Check sheet for the drawn part. Datum: minimum x, y, z corner. Units: mm. A direction names the side the tool comes from. Coordinates: 2 decimals unless noted, no trailing zeros. Loops run counter-clockwise (first coordinate to the right, second up) from the corner with the lowest first, then second, coordinate; pieces in that order, holes last. Notation, with made-up numbers: M 41.5,-3.75 L 65.5,-3.75 A26 cw 65.5,24.25 Z; hole C -3,-16.5 d5. An arc over 180 degrees is marked long. Answer as CSV lines item,"result". Start each with the question number.
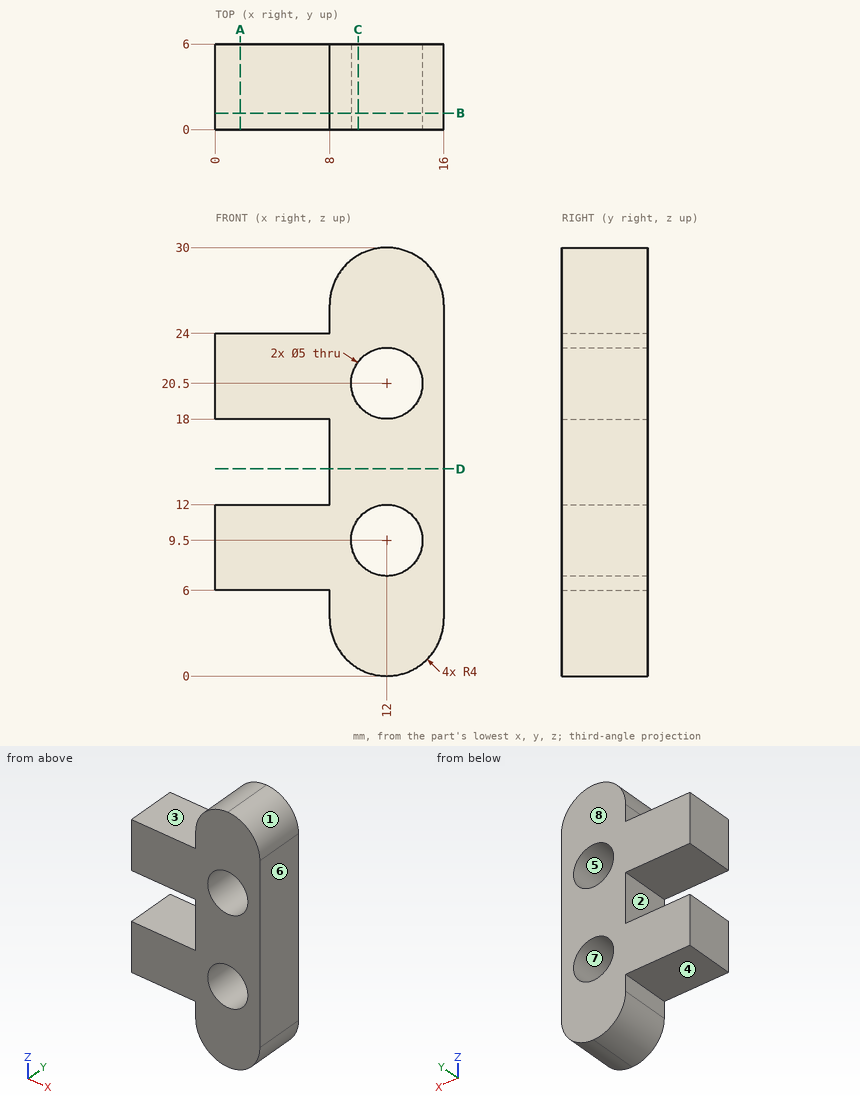
Item 1: Sectioned sample at C-C, the plane x = 10. Record the boundary of the cut face in (y, z).
Item 2: Go/stop test with flat-tipped pins: pin 1 (1.5 mm diameter, centred on y = 4.5, z = 4.5, fed in from -X); pin 2 (3 mm diameter, centred on x = 4.5, y = 1.5, fed in from +Z); pin 3 (3 mm diameter, centred on x = 5.5, y = 1.5, fed in from -Z). Record where each tip stops, or that it passes through.
Item 3: Set-up check for the marked faces 1, 2, 3 and 4: record each of +Z, -Z, +X, -X, +Y, -Y from which the full face is reachable in a straight line by a thin tool's end or side.
Item 4: Sectioned sample at B-B, the plane y = 1.15. Give the number of separate pieces and of enclosed holes in the cut face, and give its area (3 significant figures).
Item 5: Sectioned sample at D-D, the plane z = 14.5. Record the boundary of the cut face in (x, y).
Item 6: Release check for a two-part mould opening along X. For the marked faces 5, 6, 7 and 8 record: released by +X, released by -X, zero draft, split by the parting line, or undercut.
Item 7: Sectioned sample at A-A, the plane x = 1.75. Record the boundary of the cut face in (y, z).
Item 8: Material ranges on line 1 (Z direction, x = 2.75, y = 5); line 2 (X direction, y = 1.55, z = 20.5); line 3 (Z direction, x = 10, y = 1.3), recorded low to high. Write a range as from..to.
Reply:
1,outline,"M 0,0.54 L 6,0.54 L 6,8 L 0,8 Z; M 0,11 L 6,11 L 6,19 L 0,19 Z; M 0,22 L 6,22 L 6,29.46 L 0,29.46 Z"
2,pin 1,"x = 8"
2,pin 2,"z = 24"
2,pin 3,"z = 6"
3,face 1,"+Z, +X, +Y, -Y"
3,face 2,"-X, +Y, -Y"
3,face 3,"+Z, -X, +Y, -Y"
3,face 4,"-Z, -X, +Y, -Y"
4,separate pieces,"1"
4,enclosed holes,"2"
4,area,"283 mm²"
5,outline,"M 8,0 L 16,0 L 16,6 L 8,6 Z"
6,face 5,"undercut"
6,face 6,"released by +X"
6,face 7,"undercut"
6,face 8,"zero draft"
7,outline,"M 0,6 L 6,6 L 6,12 L 0,12 Z; M 0,18 L 6,18 L 6,24 L 0,24 Z"
8,line 1,"6..12, 18..24"
8,line 2,"0..9.5, 14.5..16"
8,line 3,"0.54..8, 11..19, 22..29.46"
